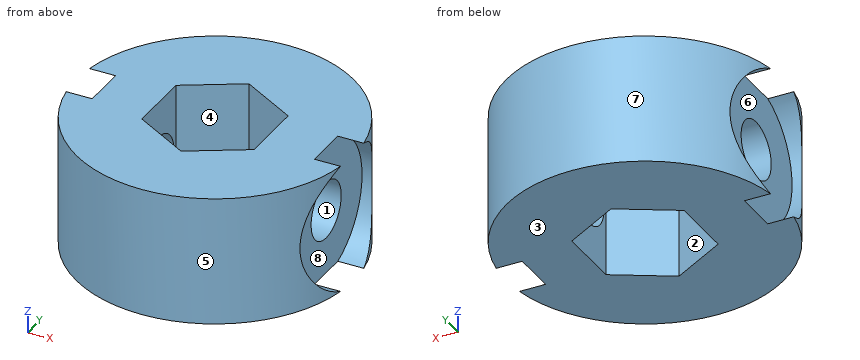
from build123d import *

# Parameters (mm, degrees)
SKETCH1_R               = 7.5
BOSS_EXTRUDE2_DEPTH     = 7
CUT_EXTRUDE1_DEPTH      = 7.5
CUT_EXTRUDE1_DEPTH_BACK = 7.5
SKETCH2_R               = 1.55
SKETCH4_R               = 3.7
CUT_EXTRUDE2_DEPTH      = 4
CUT_EXTRUDE3_START      = -4
SKETCH5_R               = 3.7
CUT_EXTRUDE3_DEPTH      = 4


with BuildPart() as part:
    # Sketch1 → Boss-Extrude2 (new body)
    with BuildSketch(Plane.XY):
        Circle(SKETCH1_R)
        Polygon((-3.031088913, 1.75), (0, 3.5), (3.031088913, 1.75), (3.031088913, -1.75), (0, -3.5), (-3.031088913, -1.75), align=None, mode=Mode.SUBTRACT)
    extrude(amount=BOSS_EXTRUDE2_DEPTH)

    # Sketch2 → Cut-Extrude1 (cut, two sides: drawn at the far end of the back side and taken through both)
    with BuildSketch(Plane.ZY.offset(-CUT_EXTRUDE1_DEPTH_BACK)):
        with Locations(Location((3.5, 0, 0), (0, 0, 180))):
            Circle(SKETCH2_R)
    extrude(amount=CUT_EXTRUDE1_DEPTH + CUT_EXTRUDE1_DEPTH_BACK, mode=Mode.SUBTRACT)

    # Sketch4 → Cut-Extrude2 (cut)
    with BuildSketch(Plane.ZY.offset(6)):
        with Locations((3.5, 0)):
            Circle(SKETCH4_R)
    extrude(amount=CUT_EXTRUDE2_DEPTH, mode=Mode.SUBTRACT)

    # Sketch5 → Cut-Extrude3 (cut)
    with BuildSketch(Plane.ZY.offset(-6).offset(CUT_EXTRUDE3_START)):
        with Locations((3.5, 0)):
            Circle(SKETCH5_R)
    extrude(amount=CUT_EXTRUDE3_DEPTH, mode=Mode.SUBTRACT)


solid = part.part
Model file for the job. Use its own axes, mm. Face numbers are marked on the shaded views. A direction names the side the tool comes from. Give positions to 0.01 mm unless a question says otherwise; leave off trailing zeros. Loops run counter-clockwise (first coordinate to the right, second up) from the corner with the lowest first, then second, coordinate; pieces in that order, holes last.
1) Saw through at C-C (z = 3.5). Write the cut outline in (x, y).
2) Tool access for the marked faces 4, 5, 6, 7 and 8: list every direction of +Z, -Z, +X, -X, +Y, -Y with a clear straight run to the whole face (end or side of a thin tool).
3) Saw through at A-A (y = 0). Write the cut outline in (x, z), plus the area to 3 significant figures.
4) Saw through at D-D (x = -4.5). Write the cut outline in (y, z).
5) Saw through at B-B (x = -2.25). Write the cut outline in (y, z).
6) Pull direction Z, two halves, no side cores. Call the marked faces 1, 2 and 3: +Z half, -Z half, draft (parallel to the pull), parting line (faces both ways), or undercut.
7) Flat gauge pins, fed straight in: pin 1 Ø1 at (y, z) = (-0.5, 4.5) entering from +X; pin 2 Ø1.5 at (y, z) = (-3.5, 3.5) entering from -X; pin 3 Ø8 at (x, y) = (-0.5, 6) entering from -Z; pin 4 Ø3 at (y, z) = (0.5, 4) entering from -X. Where does each tip first touch, or does it go through?
8) Wall check: line 1 (X direction, y = -0.5, z = 5); line 2 (Y direction, x = -6.25, z = 2); line 3 (X direction, y = -2.5, z = 3.75). Give the ranges that are in metal, low to high.
Answer block:
1. outline: (-6.52, -3.7) arc R7.5 ccw to (6.52, -3.7) - (6, -3.7) - (6, -1.55) - (3.03, -1.55) - (3.03, -1.75) - (0, -3.5) - (-3.03, -1.75) - (-3.03, -1.55) - (-6, -1.55) - (-6, -3.7) - close; (-6.52, 3.7) - (-6, 3.7) - (-6, 1.55) - (-3.03, 1.55) - (-3.03, 1.75) - (0, 3.5) - (3.03, 1.75) - (3.03, 1.55) - (6, 1.55) - (6, 3.7) - (6.52, 3.7) arc R7.5 ccw to start
2. face 4: +Z, -Z
2. face 5: +Z, -Z, -Y
2. face 6: -X
2. face 7: +Z, -Z, +Y
2. face 8: +X
3. outline: (-6, 0) - (-3.03, 0) - (-3.03, 1.95) - (-6, 1.95) - close; (-6, 5.05) - (-3.03, 5.05) - (-3.03, 7) - (-6, 7) - close; (3.03, 0) - (6, 0) - (6, 1.95) - (3.03, 1.95) - close; (3.03, 5.05) - (6, 5.05) - (6, 7) - (3.03, 7) - close
3. area: 23.2 mm2
4. outline: (-6, 0) - (6, 0) - (6, 7) - (-6, 7) - close; hole circle Ø3.1 at (0, 3.5)
5. outline: (-7.15, 0) - (-2.2, 0) - (-2.2, 7) - (-7.15, 7) - close; (2.2, 0) - (7.15, 0) - (7.15, 7) - (2.2, 7) - close
6. face 1: undercut
6. face 2: draft
6. face 3: -Z half
7. pin 1: stops at x = 6
7. pin 2: stops at x = -6.57
7. pin 3: stops at z = 0
7. pin 4: stops at x = -6
8. line 1: x = -6 to -3.03, 3.03 to 6
8. line 2: y = -4.15 to -3.38, 3.38 to 4.15
8. line 3: x = -6 to -1.73, 1.73 to 6
